Model file for the job. Use its own axes, mm. A direction names the side the tool comes from. Coordinates: 2 decimals unless noted, no trailing zeros. Write each loop counter-clockwise with the first axis right and the second up, starting at its lowest first coordinate (ties: lowest second). Pieces come first, ordered by that corner, then holes. Notation, with made-up numbers: M 49.5,86.25 L 60.5,86.25 A31 cw 60.5,121.25 Z; hole C -27,53.25 d3. An arc over 180 degrees is marked long. One line per question, with ' | ' between items. Start each with the question number.
(1) Tool access for faces 1 (the face through (1, -310.355, 139)), 2 (the face through (0, -300, 145)), 3 (the face through (1, -294, 146.133)): list every direction of +Z, -Z, +X, -X, +Y, -Y with a clear straight run to the whole face (end or side of a thin tool).
(2) Flat gauge pins, fed straight in: pin 1 Ø1.4 at (x, y) = (2, -293) entering from -Z; pin 2 Ø1.5 at (x, z) = (1.5, 140.5) entering from +Y; pin 3 Ø1.5 at (x, z) = (1, 134.5) entering from -Y; pin 4 Ø4 at (y, z) = (-303.5, 134.5) entering from -X. Where does each tip first touch, or does it go through?
(3) Wall check: probe 1 along Z at (x, y) = (1.2, -302.75); probe 2 along Y at (x, z) = (1.5, 141); probe 3 along Y at (x, z) = (0.35, 136). Give the ranges that are in metal, low to high.
(4) Cut at D-D (y = -293.5). Write the cut outline in (x, z).
(5) Cut at B-B (y = -299.75). Write the cut outline in (x, z).
(6) Cut at A-A (z = 141.5). Write the cut outline in (x, y).
(7) Two-plate mould, pull along Y, no slides. Class faces 4 (the face through (1.48, -305.55, 143.84)), 5 (the face through (1, -292.131, 148)), 6 (the face through (1, -303, 132.633)): +Y half, -Y half, draft (parallel to the pull), parting line (faces both ways), or undercut.
(8) Cut at C-C (x = 0.95). Write the cut outline in (y, z).
from build123d import *

# Parameters (mm, degrees)
F0_W     = 15.5
F0_H     = 13.5
F0_R     = 4
F1_DEPTH = 3


with BuildPart() as f1:
    # F0 (on Right) → F1 (new body)
    with BuildSketch(Plane.YZ):
        Polygon((-313.131073, 146.133296), (-310.35515, 146.133296), (-294.85515, 146.133296), (-292.131073, 146.133296), (-292.131073, 149.633296), (-313.131073, 149.633296), align=None)
        with Locations((-302.60515, 139.383296)):
            Rectangle(F0_W, F0_H)
        with Locations((-302.60515, 141.133296)):
            Circle(F0_R, mode=Mode.SUBTRACT)
    extrude(amount=F1_DEPTH)


solid = f1.part
Filled in:
1) face 1: -Z, +X, -X, -Y | face 2: +Z, -Z, -X, +Y, -Y | face 3: -Z, +X, -X, +Y
2) pin 1: z = 146.13 | pin 2: y = -294.86 | pin 3: y = -310.36 | pin 4: x = 0
3) probe 1: 132.63 to 137.14, 145.13 to 149.63 | probe 2: -310.36 to -306.6, -298.61 to -294.86 | probe 3: -310.36 to -294.86
4) outline: M 0,146.13 L 3,146.13 L 3,149.63 L 0,149.63 Z
5) outline: M 0,132.63 L 3,132.63 L 3,138.33 L 0,138.33 Z; M 0,143.93 L 3,143.93 L 3,149.63 L 0,149.63 Z
6) outline: M 0,-310.36 L 3,-310.36 L 3,-306.59 L 0,-306.59 Z; M 0,-298.62 L 3,-298.62 L 3,-294.86 L 0,-294.86 Z
7) face 4: undercut | face 5: +Y half | face 6: draft
8) outline: M -313.13,146.13 L -310.36,146.13 L -310.36,132.63 L -294.86,132.63 L -294.86,146.13 L -292.13,146.13 L -292.13,149.63 L -313.13,149.63 Z; hole C -302.61,141.13 d8
